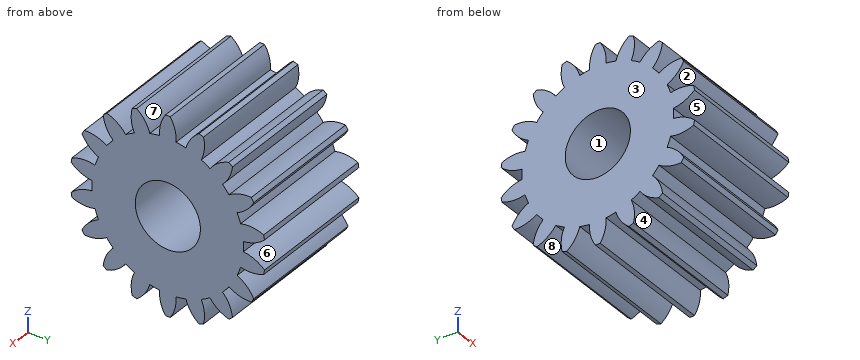
```python
from build123d import *

# Parameters (mm, degrees)
BASPROSKE_W        = 8
BASPROSKE_H        = 6
TOOTHCUT_DEPTH     = 12.66190379
TEETHCUTS_COUNT    = 18
TEETHCUTS_ANGLE    = 340
BORSKE_R           = 0.5
BORE_DEPTH         = 50.0000508
SKETCH1_R          = 2
CUT_EXTRUDE1_DEPTH = 12.627390673


with BuildPart() as part:
    # BasProSke → Base-Revolve (revolve)
    with BuildSketch(Plane(origin=(0, 0, 0), x_dir=(1, 0, 0), z_dir=(0, 1, 0)), mode=Mode.PRIVATE) as base_revolve_sk:
        with Locations((4, 3)):
            Rectangle(BASPROSKE_W, BASPROSKE_H)
    revolve(base_revolve_sk.sketch.rotate(Axis((-10, 0, 0), (1, 0, 0)), 180), axis=Axis((-10, 0, 0), (1, 0, 0)))

    # TooCutSke → ToothCut (cut, through all)
    with BuildSketch(Plane(origin=(0, 0, 0), x_dir=(0, 0, -1), z_dir=(1, 0, 0))):
        with BuildLine():
            ThreePointArc((0.306649621, 4.638875619), (0, 4.649), (-0.306649621, 4.638875619))
            ThreePointArc((-0.306649621, 4.638875619), (-0.498605842, 5.349852231), (-0.918258882, 5.955018538))
            ThreePointArc((-0.918258882, 5.955018538), (0, 6.0254), (0.918258882, 5.955018538))
            ThreePointArc((0.918258882, 5.955018538), (0.498605842, 5.349852231), (0.306649621, 4.638875619))
        make_face()
    toothcut = extrude(amount=TOOTHCUT_DEPTH, mode=Mode.SUBTRACT)

    # TeethCuts: ToothCut ×18 about axis
    teethcuts_axis = Axis((-10, 0, 0), (1, 0, 0))
    for i in range(1, TEETHCUTS_COUNT):
        add(toothcut.rotate(teethcuts_axis, i * TEETHCUTS_ANGLE / (TEETHCUTS_COUNT - 1)), mode=Mode.SUBTRACT)

    # BorSke → Bore (cut, symmetric)
    with BuildSketch(Plane(origin=(0, 0, 0), x_dir=(0, 0, -1), z_dir=(1, 0, 0))):
        with Locations(Location((0, 0, 0), (0, 0, 180))):
            Circle(BORSKE_R)
    extrude(amount=BORE_DEPTH, both=True, mode=Mode.SUBTRACT)

    # Sketch1 → Cut-Extrude1 (cut, through all)
    with BuildSketch(Plane(origin=(8, 0, 0), x_dir=(0, 0, -1), z_dir=(1, 0, 0))):
        Circle(SKETCH1_R)
    extrude(amount=-CUT_EXTRUDE1_DEPTH, mode=Mode.SUBTRACT)


solid = part.part
```
Geometry check sheet. Reference: the model listing, model coordinates, mm. Face numbers are marked on the shaded views. A direction names the side the tool comes from. Give positions to 0.01 mm unless a question says otherwise; leave off trailing zeros. Loops run counter-clockwise (first coordinate to the right, second up) from the corner with the lowest first, then second, coordinate; pieces in that order, holes last. Notation, with made-up numbers: M 13,-2 L 23,-2 A27 cw 23,36 Z; hole C 82.25,-35.75 d10. An arc over 180 degrees is marked long. Write item = value, one per line.
(1) Gauge pin test, flat ends, axial feed: pin 1 Ø2 at (x, z) = (4.5, 2) entering from +Y; pin 2 Ø1.5 at (x, z) = (6, -4) entering from -Y; pin 3 Ø1 at (x, z) = (4.5, 2) entering from -Y; pin 4 Ø6.5 at (y, z) = (0, 0) entering from -X. Record the tip position at first contact, or that the pin passes through.
Answer below:
pin_1 = 5.92
pin_2 = -3.97
pin_3 = -5.04
pin_4 = 0
(2) Material ranges on line 1 (Y direction, x = 5.25, z = 0); line 2 (Y direction, x = 3, z = 1.5); line 3 (Z direction, x = 6.5, y = 5.75), recorded low to high. Write a range as [from, to].
Answer below:
line_1 = [-4.65, -2], [2, 4.65]
line_2 = [-4.4, -1.32], [1.32, 4.4]
line_3 = [-1.24, -0.74], [0.74, 1.24]
(3) Sectioned sample at B-B, the plane y = -3. Record the cut outline in (x, z), plus the area to 3 significant figures.
Answer below:
outline = M 0,-4.3 L 8,-4.3 L 8,4.3 L 0,4.3 Z
area = 68.9 mm2
(4) Release check for a two-part mould opening along Y. For the marked faces 1, 2 and 3 record: released by +Y, released by -Y, zero draft, split by the parting line, or undercut.
Answer below:
face_1 = undercut
face_2 = released by -Y
face_3 = zero draft
(5) Sectioned sample at A-A, the plane z = 0. Record the cut outline in (x, y), plus the area to 3 significant figures.
Answer below:
outline = M 0,-4.65 L 8,-4.65 L 8,-2 L 0,-2 Z; M 0,2 L 8,2 L 8,4.65 L 0,4.65 Z
area = 42.4 mm2
(6) Tool access check on the marked faces 4, 5, 6, 7 and 8. Record the directions out of +Z, -Z, +X, -X, +Y, -Y that give a thin tool (end or side, any length) a straight path to the whole face; none if there is none.
Answer below:
face_4 = +X, -X
face_5 = +X, -X, -Y
face_6 = +X, -X, +Y
face_7 = +Z, +X, -X
face_8 = -Z, +X, -X
